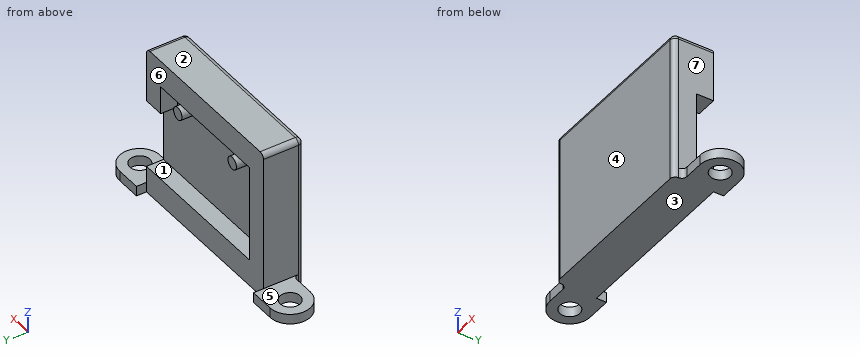
```python
from build123d import *

# Parameters (mm, degrees)
CROQUIS1_W              = 35
CROQUIS1_H              = 30
SALIENTE_EXTRUIR1_DEPTH = 8
CROQUIS2_R              = 1.25
CORTAR_EXTRUIR2_DEPTH   = 3.4
CROQUIS3_R              = 2
SALIENTE_EXTRUIR2_DEPTH = 2
REDONDEO1_R             = 1


with BuildPart() as part:
    # Croquis1 → Saliente-Extruir1 (new body)
    with BuildSketch(Plane(origin=(0, 0, 0), x_dir=(1, 0, 0), z_dir=(0, 1, 0))):
        Rectangle(CROQUIS1_W, CROQUIS1_H)
    extrude(amount=SALIENTE_EXTRUIR1_DEPTH)

    # Croquis2 → Cortar-Extruir2 (cut)
    with BuildSketch(Plane(origin=(0, 8, 0), x_dir=(1, 0, 0), z_dir=(0, 1, 0))):
        Polygon((13.25, 9.65), (17.5, 9.65), (17.5, -4.05), (13.25, -4.05), (13.25, -9.65), (-13.25, -9.65), (-13.25, 9.65), align=None)
        with Locations(Location((-8.15, -7.3, 0), (0, 0, 270))):
            Circle(CROQUIS2_R, mode=Mode.SUBTRACT)
        with Locations(Location((8.15, -7.3, 0), (0, 0, 270))):
            Circle(CROQUIS2_R, mode=Mode.SUBTRACT)
    extrude(amount=-CORTAR_EXTRUIR2_DEPTH, mode=Mode.SUBTRACT)

    # Croquis3 → Saliente-Extruir2 (add)
    # profile 1 of 2: a face of its own
    with BuildSketch(Plane(origin=(0, 0, -15), x_dir=(-1, 0, 0), z_dir=(0, 0, -1))):
        with BuildLine():
            Line((-17.5, 2), (-17.5, 10))
            Line((-17.5, 10), (-22.5, 10))
            ThreePointArc((-22.5, 10), (-26.5, 6), (-22.5, 2))
            Line((-22.5, 2), (-17.5, 2))
        make_face()
        with Locations((-22.5, 6)):
            Circle(CROQUIS3_R, mode=Mode.SUBTRACT)
    # profile 2 of 2: a face of its own
    with BuildSketch(Plane(origin=(0, 0, -15), x_dir=(-1, 0, 0), z_dir=(0, 0, -1))):
        with BuildLine():
            Line((17.5, 10), (22.5, 10))
            ThreePointArc((22.5, 10), (26.5, 6), (22.5, 2))
            Line((22.5, 2), (17.5, 2))
            Line((17.5, 2), (17.5, 10))
        make_face()
        with Locations(Location((22.5, 6, 0), (0, 0, 180))):
            Circle(CROQUIS3_R, mode=Mode.SUBTRACT)
    extrude(amount=-SALIENTE_EXTRUIR2_DEPTH)

    # Redondeo1
    redondeo1_edges = [part.edges().sort_by_distance(p)[0] for p in [
        (17.5, 2, -14),
        (17.5, 0, 0),
        (0, 0, 15),
        (-17.5, 0, 0),
        (-17.5, 2, -14),
        (-17.5, 4, 15),
        (17.5, 4, 15),
    ]]
    fillet(redondeo1_edges, radius=REDONDEO1_R - 0.0001)  # a hair under: the kernel refuses the full size


solid = part.part
```
Design review of the part built by this model. Coordinates are the model's own, in mm. Face numbers are marked on the shaded views. A direction names the side the tool comes from. Round coordinates to 2 decimals unless told otherwise and drop trailing zeros. Write each loop counter-clockwise with the first axis right and the second up, starting at its lowest first coordinate (ties: lowest second). Pieces come first, ordered by that corner, then holes.
Item 1: The part is to be moulded in two halves that separate along Z. For the marked faces 1, 2 and 3, say which applies: +Z half, -Z half, draft (parallel to the pull), parting line (faces both ways), or undercut.
Item 2: We need section D-D on y = 8.5. Write out the cut boundary in (x, z).
Item 3: For the marked faces 4, 5, 6 and 7, list the 3-axis set-ups (+Z, -Z, +X, -X, +Y, -Y) from which the entire face can be reached by the end or side of a thin tool; tool diameter is ignored.
Item 4: Clearance check with flat-ended pins moving along their axes: pin 1 Ø2.5 at (x, y) = (20, 6.5) entering from +Z; pin 2 Ø1 at (x, z) = (20, -13.5) entering from -Y; pin 3 Ø1 at (y, z) = (9.5, -14) entering from -X. State where each tip first meets the part, or that it passes through.
Item 5: We need section B-B on x = 0.5. Write out the cut boundary in (y, z).
Item 6: For probe 1 along Z at (x, y) = (0.5, 5); probe 2 along Y at (x, z) = (22.5, -14.5); probe 3 along Z at (x, y) = (8.5, 5), list the stretches that pass through material, from the lowest coordinate up.
Item 7: We need section C-C on z = 0.75. Write out the cut boundary in (x, y), and give its area (3 significant figures).
Item 8: We need section A-A on y = 6. Write out the cut boundary in (x, z), and give its area (3 significant figures).
Returned:
1. face 1: undercut
1. face 2: +Z half
1. face 3: -Z half
2. outline: (-25.62, -15) - (-17.5, -15) - (-17.5, -13) - (-25.62, -13) - close; (17.5, -15) - (25.62, -15) - (25.62, -13) - (17.5, -13) - close
3. face 4: +Z, -Z, +X, -X, -Y
3. face 5: +Z, -X, +Y, -Y
3. face 6: +Z, -Z, +Y
3. face 7: +Z, +X, +Y, -Y
4. pin 1: stops at z = -13
4. pin 2: stops at y = 2
4. pin 3: stops at x = -25.15
5. outline: (0, -15) - (8, -15) - (8, -9.65) - (4.6, -9.65) - (4.6, 9.65) - (8, 9.65) - (8, 15) - (1, 15) arc R1 ccw to (0, 14) - close
6. probe 1: z = -15 to -9.65, 9.65 to 15
6. probe 2: y = 2 to 4, 8 to 10
6. probe 3: z = -15 to -9.65, 6.1 to 8.5, 9.65 to 15
7. outline: (-17.5, 1) arc R1 ccw to (-16.5, 0) - (16.5, 0) arc R1 ccw to (17.5, 1) - (17.5, 4.6) - (-13.25, 4.6) - (-13.25, 8) - (-17.5, 8) - close
7. area: 175 mm2
8. outline: (-26.5, -15) - (-24.5, -15) - (-24.5, -13) - (-26.5, -13) - close; (-20.5, -15) - (20.5, -15) - (20.5, -13) - (17.5, -13) - (17.5, -9.65) - (-13.25, -9.65) - (-13.25, 9.65) - (13.25, 9.65) - (13.25, 4.05) - (17.5, 4.05) - (17.5, 14) arc R1 ccw to (16.5, 15) - (-16.5, 15) arc R1 ccw to (-17.5, 14) - (-17.5, -13) - (-20.5, -13) - close; circle Ø2.5 at (-8.15, 7.3); circle Ø2.5 at (8.15, 7.3); (24.5, -15) - (26.5, -15) - (26.5, -13) - (24.5, -13) - close
8. area: 510 mm2
